```python
from build123d import *

# Parameters (mm, degrees)
F0_W     = 12
F0_H     = 50
F0_R     = 3
F1_DEPTH = 5
F2_R     = 5.99999
F3_DEPTH = 10


# Not quite as in the source:
# - a fillet or chamfer is up to 0.001 mm smaller than in the source, because OpenCascade refuses the exact size


with BuildPart() as f1:
    # F0 (on Top) → F1 (new body)
    with BuildSketch(Plane.XY):
        with Locations((-0.8723753854, -8.5783358663)):
            Rectangle(F0_W, F0_H)
        with Locations((-0.8723753854, -27.5783358663)):
            Circle(F0_R, mode=Mode.SUBTRACT)
        with Locations((-0.8723753854, 10.4216641337)):
            Circle(F0_R, mode=Mode.SUBTRACT)
    extrude(amount=F1_DEPTH)

    # F2 (radius 6 in the source; OpenCascade refuses exactly that, so slightly less here)
    f2_edges = [f1.edges().sort_by_distance(p)[0] for p in [
        (-6.872375, 16.421664, 2.5),
        (5.127625, 16.421664, 2.5),
        (5.127625, -33.578336, 2.5),
        (-6.872375, -33.578336, 2.5),
    ]]
    fillet(f2_edges, radius=F2_R)

    # F0 (on Top) → F3 (join)
    with BuildSketch(Plane.XY):
        with Locations((-0.8723753854, 10.4216641337)):
            Circle(F0_R)
    extrude(amount=F3_DEPTH)


solid = f1.part
```
Input: part model. Units: mm. Frame: model coordinates. A direction names the side the tool comes from. Give positions to 0.01 mm unless a question says otherwise; leave off trailing zeros. Order: outer loops, then holes, each group sorted by start corner. A loop starts at its lowest first (then second) coordinate and runs counter-clockwise, first axis right, second up. Notation, with made-up numbers: (76, 41.25) - (120, 41.25) arc R36 ccw to (120, 77.25) - close; hole circle Ø2 at (-39, 72). An arc over 180 degrees is marked (long way). Use a Markdown table: item, result.
(1) Line query: line 1 (Y direction, x = -1, z = 3.75); line 2 (Z direction, x = -1.5, y = -18); line 3 (Y direction, x = 1, z = 4). Output: solid intervals per line, ascending. Write a range as from..to.
Computed values:
| item | result |
|---|---|
| line 1 | y = -33.58..-30.58, -24.58..16.42 |
| line 2 | z = 0..5 |
| line 3 | y = -33.28..-29.92, -25.23..16.12 |
(2) Section query D-D (z = 8.25). Output: boundary loops of the cut face in (x, y), then the cut area to 3 significant figures.
Computed values:
| item | result |
|---|---|
| outline | circle Ø6 at (-0.87, 10.42) |
| area | 28.3 mm2 |
(3) Draft query along Y for faces 1 (the cylindrical face through (-1.263, -24.604, 2.465)), 2 (the cylindrical face through (3.32, -31.87, 2.54)), 3 (the flat face through (-1, -8, 5)). Return one class per face: released by +Y, released by -Y, zero draft, split by the parting line, or undercut.
Computed values:
| item | result |
|---|---|
| face 1 | undercut |
| face 2 | released by -Y |
| face 3 | zero draft |
(4) Section query A-A (x = 1.25). Output: boundary loops of the cut face in (y, z).
Computed values:
| item | result |
|---|---|
| outline | (-33.19, 0) - (-29.7, 0) - (-29.7, 5) - (-33.19, 5) - close; (-25.46, 0) - (16.03, 0) - (16.03, 5) - (12.54, 5) - (12.54, 10) - (8.3, 10) - (8.3, 5) - (-25.46, 5) - close |
(5) Access query for faces 4 (the cylindrical face through (-1.263, 13.396, 7.465)), 5 (the cylindrical face through (-5.161, -31.774, 2.535)). Directions: +Z, -Z, +X, -X, +Y, -Y. A direction counts if a zero-diameter tool reaches every point of the face in a straight line with its end or side. Return the directions, or none.
Computed values:
| item | result |
|---|---|
| face 4 | +Z |
| face 5 | +Z, -Z, -X, -Y |
(6) Section query C-C (y = 9). Output: boundary loops of the cut face in (x, z).
Computed values:
| item | result |
|---|---|
| outline | (-6.87, 0) - (5.13, 0) - (5.13, 5) - (1.77, 5) - (1.77, 10) - (-3.51, 10) - (-3.51, 5) - (-6.87, 5) - close |
(7) Pin query (flat end, axial travel): pin 1 (1.5 mm diameter, centred on y = 11, z = 7.5, fed in from +X). Return the tip coordinate at first contact, or that it passes through.
Computed values:
| item | result |
|---|---|
| pin 1 | stops at x = 2.13 |
